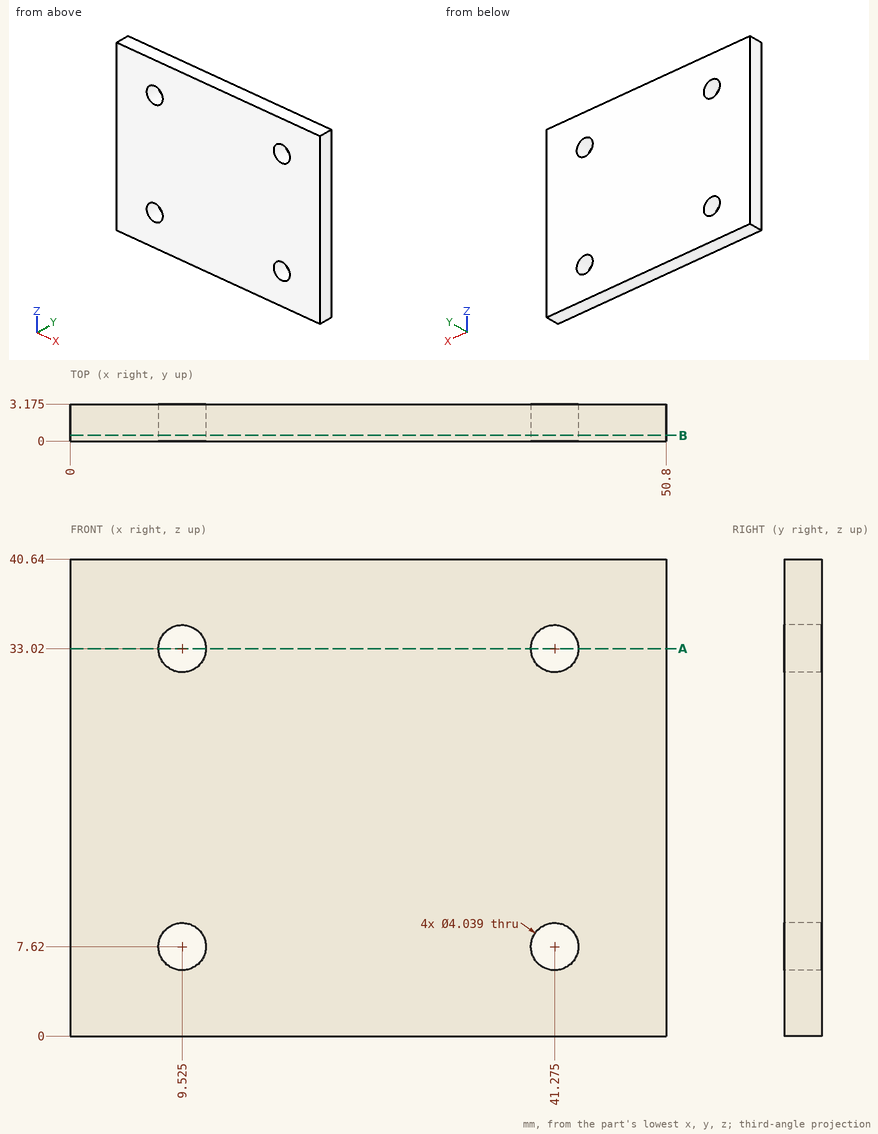
Here's the drawing with two shaded views (mm, measured from the low corner). I have some questions. Give positions to 0.01 mm unless a question says otherwise; leave off trailing zeros. Write each loop counter-clockwise with the first axis right and the second up, starting at its lowest first coordinate (ties: lowest second). Pieces come first, ordered by that corner, then holes. Notation, with made-up numbers: (62, 7.25) - (114, 7.25) arc R16 cw to (114, 18.25) - close; hole circle Ø7 at (-7.75, -16.75). An arc over 180 degrees is marked (long way). One line per item, written item: value. Start each with the question number.
Item 1: Please list where these lines run through material, in increasing order: line 1 (X direction, y = 1.1, z = 33.02) (1 decimal); line 2 (Z direction, x = 9.5, y = 1.9); line 3 (X direction, y = 0.75, z = 6). Write a range as from..to.
Item 2: Imagine slicing it at B-B, the plane y = 0.5. List the corners of the cut face in (x, z) for me (1 decimal).
Item 3: Imagine slicing it at A-A, the plane z = 33.02. List the corners of the cut face in (x, y) for me (1 decimal), and give its area (3 significant figures).
Geometry says:
1. line 1: 0..7.5, 11.5..39.3, 43.3..50.8
1. line 2: 0..5.6, 9.64..31, 35.04..40.64
1. line 3: 0..8.32, 10.73..40.07, 42.48..50.8
2. outline: (0, 0) - (50.8, 0) - (50.8, 40.6) - (0, 40.6) - close; hole circle Ø4 at (9.5, 7.6); hole circle Ø4 at (9.5, 33); hole circle Ø4 at (41.3, 7.6); hole circle Ø4 at (41.3, 33)
3. outline: (0, 0) - (7.5, 0) - (7.5, 3.2) - (0, 3.2) - close; (11.5, 0) - (39.3, 0) - (39.3, 3.2) - (11.5, 3.2) - close; (43.3, 0) - (50.8, 0) - (50.8, 3.2) - (43.3, 3.2) - close
3. area: 136 mm^2
